Geometry check sheet. Reference: the model listing, model coordinates, mm. A direction names the side the tool comes from. Give positions to 0.01 mm unless a question says otherwise; leave off trailing zeros. Write each loop counter-clockwise with the first axis right and the second up, starting at its lowest first coordinate (ties: lowest second). Pieces come first, ordered by that corner, then holes. Notation, with made-up numbers: (73.5, 38) -> (127.5, 38) arc R14 cw to (127.5, 43) -> close; hole circle Ø2 at (-33.75, 58). An arc over 180 degrees is marked (long way). Write item = value, one per line. Start each with the question number.
1. Cross-section at D-D, the plane x = 1.25. Record the cut outline in (y, z), plus the area to 3 significant figures.
2. Cross-section at B-B, the plane x = -2.5. Record the cut outline in (y, z).
3. Cross-section at A-A, the plane z = -0.9. Record the cut outline in (x, y).
4. Set-up check for faces 1 (the flat face through (1.753, 4, 0)), 2 (the flat face through (0, 2, -1.651)): record each of +Z, -Z, +X, -X, +Y, -Y from which the full face is reachable in a straight line by a thin tool's end or side.
5. Cross-section at C-C, the plane z = -0.3. Record the cut outline in (x, y), plus the area to 3 significant figures.
6. Thickness scan on line 1 along Y through (x, z) = (2.5, -0.3); line 2 along X through (y, z) = (4, 0.2); line 3 along Y through (x, z) = (-2.5, 1.4). Record the ranges inside material, lowest first.
7. Mould release check, pull along Z, two halves, no side actions. Record for faces 3 (the flat face through (1, 4, 0.749)), 4 (the flat face through (1, 4, -0.749)), 5 (the flat face through (0.254, 4, 0)): pulls with the +Z half, pulls with the -Z half, needs draft (parallel to the pull), parting line crosses it, or undercut.
8. Depth check by flat-ended pin: P1, Ø1, axis at x = -1.5, z = 0, coming from the +Y side. Enter the tip coordinate at first touch or a pass-through.
```python
from build123d import *

# Parameters (mm, degrees)
SKETCH1_W               = 8.9916
SKETCH1_H               = 3.302
BOSS_EXTRUDE1_DEPTH     = 3.5052
SKETCH2_W               = 1.4986
SKETCH2_H               = 1.4986
BOSS_EXTRUDE2_DEPTH     = 2.0066
SKETCH3_W               = 0.6096
SKETCH3_H               = 0.3048
BOSS_EXTRUDE3_DEPTH     = 2.9972
LPATTERN1_COUNT         = 3
LPATTERN1_PITCH         = 2.4892
MIRROR1_COPY_1_SKETCH_W = 0.6096
MIRROR1_COPY_1_SKETCH_H = 0.3048
MIRROR1_COPY_1_DEPTH    = 2.9972
MIRROR1_COPY_2_SKETCH_W = 0.6096
MIRROR1_COPY_2_SKETCH_H = 0.3048
MIRROR1_COPY_2_DEPTH    = 2.9972
FILLET1_R               = 0.5


with BuildPart() as part:
    # Sketch1 → Boss-Extrude1 (new body)
    with BuildSketch(Plane(origin=(0, 0, 0), x_dir=(1, 0, 0), z_dir=(0, 1, 0))):
        Rectangle(SKETCH1_W, SKETCH1_H)
    extrude(amount=BOSS_EXTRUDE1_DEPTH)

    # Sketch2 → Boss-Extrude2 (add)
    with BuildSketch(Plane(origin=(0, 3.5052, 0), x_dir=(1, 0, 0), z_dir=(0, 1, 0))):
        with Locations((1.0033, 0)):
            Rectangle(SKETCH2_W, SKETCH2_H)
    extrude(amount=BOSS_EXTRUDE2_DEPTH)

    # Sketch3 → Boss-Extrude3 (add)
    with BuildSketch(Plane.XZ):
        with Locations((2.4892, 1.4986)):
            Rectangle(SKETCH3_W, SKETCH3_H)
    boss_extrude3 = extrude(amount=BOSS_EXTRUDE3_DEPTH)

    # LPattern1: Boss-Extrude3 ×3
    with Locations(*[(-i * LPATTERN1_PITCH, 0, 0) for i in range(1, LPATTERN1_COUNT)]):
        add(boss_extrude3)

    # Mirror1: Boss-Extrude3 across plane
    add(boss_extrude3.mirror(Plane.XY))

    # Mirror1 copy 1 sketch → Mirror1 copy 1 (add)
    with BuildSketch(Plane(origin=(-2.4892, 0, 0), x_dir=(1, 0, 0), z_dir=(0, -1, 0))):
        with Locations((2.4892, -1.4986)):
            Rectangle(MIRROR1_COPY_1_SKETCH_W, MIRROR1_COPY_1_SKETCH_H)
    extrude(amount=MIRROR1_COPY_1_DEPTH)

    # Mirror1 copy 2 sketch → Mirror1 copy 2 (add)
    with BuildSketch(Plane(origin=(-4.9784, 0, 0), x_dir=(1, 0, 0), z_dir=(0, -1, 0))):
        with Locations((2.4892, -1.4986)):
            Rectangle(MIRROR1_COPY_2_SKETCH_W, MIRROR1_COPY_2_SKETCH_H)
    extrude(amount=MIRROR1_COPY_2_DEPTH)

    # Fillet1
    fillet1_edges = [part.edges().sort_by_distance(p)[0] for p in [
        (4.4958, 3.5052, 0),
        (-4.4958, 3.5052, 0),
    ]]
    fillet(fillet1_edges, radius=FILLET1_R)


solid = part.part
```
Answers:
q1.outline = (0, -1.65) -> (3.51, -1.65) -> (3.51, -0.75) -> (5.51, -0.75) -> (5.51, 0.75) -> (3.51, 0.75) -> (3.51, 1.65) -> (0, 1.65) -> close
q1.area = 14.6 mm^2
q2.outline = (-3, -1.65) -> (3.51, -1.65) -> (3.51, 1.65) -> (-3, 1.65) -> (-3, 1.35) -> (0, 1.35) -> (0, -1.35) -> (-3, -1.35) -> close
q3.outline = (-4.5, 0) -> (4.5, 0) -> (4.5, 3.01) arc R0.5 ccw to (4, 3.51) -> (-4, 3.51) arc R0.5 ccw to (-4.5, 3.01) -> close
q4.face_1 = +Z, -Z, +X, +Y
q4.face_2 = -Z, +X, -X, +Y, -Y
q5.outline = (-4.5, 0) -> (4.5, 0) -> (4.5, 3.01) arc R0.5 ccw to (4, 3.51) -> (1.75, 3.51) -> (1.75, 5.51) -> (0.25, 5.51) -> (0.25, 3.51) -> (-4, 3.51) arc R0.5 ccw to (-4.5, 3.01) -> close
q5.area = 34.4 mm^2
q6.line_1 = 0 to 3.51
q6.line_2 = 0.25 to 1.75
q6.line_3 = -3 to 3.51
q7.face_3 = pulls with the +Z half
q7.face_4 = pulls with the -Z half
q7.face_5 = needs draft
q8.P1 = 3.51
